Verification items for the finished model (mm, model axes). Give positions to 0.01 mm unless a question says otherwise; leave off trailing zeros. Loops run counter-clockwise (first coordinate to the right, second up) from the corner with the lowest first, then second, coordinate; pieces in that order, holes last. Notation, with made-up numbers: (48, -39.75) - (60, -39.75) arc R22 cw to (60, -30.75) - close; hole circle Ø4 at (-6.75, 1.5). An arc over 180 degrees is marked (long way). One line per question, with ' | ' between items. Start each with the question number.
1. Section check A-A, the plane z = 2.75. Enter the section's corners in (x, y).
2. Mould release check, pull along X, two halves, no side actions. Record for faces 1 (the face through (0.27, 1.22, 2.03)), 2 (the face through (4.594, -3.219, 3.512)), 3 (the face through (0, 2, 0)), 4 (the face through (-4.594, 3.219, 3.512)): +X half, -X half, draft (parallel to the pull), parting line (faces both ways), or undercut.
3. Thickness scan on line 1 along Y through (x, z) = (0, 1.45); line 2 along X through (y, z) = (0.5, 2.75); line 3 along Y through (x, z) = (-5, 1.75). Record the ranges inside material, lowest first. Write a range as from..to.
4. Section check D-D, the plane x = 3.5. Enter the section's corners in (y, z), then the cut area to 3 significant figures.
5. Section check C-C, the plane y = -1.75. Enter the section's corners in (x, z).
6. Section check B-B, the plane z = 5.75. Enter the section's corners in (x, y), then the cut area to 3 significant figures.
7. Depth check by flat-ended pin: pin 1 Ø2 at (x, y) = (0, 0) entering from -Z; pin 2 Ø1.5 at (y, z) = (2.5, 4.5) entering from +X. Enter the tip coordinate at first touch or a pass-through.
from build123d import *

# Parameters (mm, degrees)
SKETCH1_W                       = 12.7
SKETCH1_H                       = 12.7
BOSS_EXTRUDE1_DEPTH             = 6.928
TAP_DRILL_FOR_M3X0_5_TAP3_D     = 2.5
TAP_DRILL_FOR_M3X0_5_TAP3_DEPTH = 4
TAP_DRILL_FOR_M3X0_5_TAP3_TIP   = 0.751075774
CUT_EXTRUDE1_DEPTH              = 12.342053782
MIRROR2_COPY_1_DEPTH            = 12.342053782


with BuildPart() as part:
    # Sketch1 → Boss-Extrude1 (new body)
    with BuildSketch(Plane.XY):
        Rectangle(SKETCH1_W, SKETCH1_H)
    extrude(amount=BOSS_EXTRUDE1_DEPTH)

    # Tap Drill for M3x0.5 Tap3
    with Locations(Plane(origin=(0, 0, 0), x_dir=(1, 0, 0), z_dir=(0, 0, -1))):
        with Locations((0, 0)):
            Hole(TAP_DRILL_FOR_M3X0_5_TAP3_D / 2, depth=TAP_DRILL_FOR_M3X0_5_TAP3_DEPTH)
            with Locations((0, 0, -(TAP_DRILL_FOR_M3X0_5_TAP3_DEPTH + TAP_DRILL_FOR_M3X0_5_TAP3_TIP / 2))):  # 118° drill point
                Cone(0, TAP_DRILL_FOR_M3X0_5_TAP3_D / 2, TAP_DRILL_FOR_M3X0_5_TAP3_TIP, mode=Mode.SUBTRACT)

    # Sketch8 → Cut-Extrude1 (cut, symmetric)
    with BuildSketch(Plane.XY):
        Polygon((-16.943244885, 42.69979937), (2.886, 6.35), (6.35, 0), (26.179244885, -36.34979937), (98.878843624, 3.308690399), (55.756353855, 82.358289139), align=None)
    cut_extrude1 = extrude(amount=CUT_EXTRUDE1_DEPTH, both=True, mode=Mode.SUBTRACT)

    # Mirror1: Cut-Extrude1 across plane
    add(cut_extrude1.mirror(Plane.ZX), mode=Mode.SUBTRACT)

    # Mirror2: Cut-Extrude1 across plane
    add(cut_extrude1.mirror(Plane(origin=(0, 0, 0), x_dir=(0, 0, 1), z_dir=(1, 0, 0))), mode=Mode.SUBTRACT)

    # Mirror2 copy 1 sketch → Mirror2 copy 1 (cut, symmetric)
    with BuildSketch(Plane(origin=(0, 0, 0), x_dir=(-1, 0, 0), z_dir=(0, 0, 1))):
        Polygon((-16.943244885, 42.69979937), (2.886, 6.35), (6.35, 0), (26.179244885, -36.34979937), (98.878843624, 3.308690399), (55.756353855, 82.358289139), align=None)
    extrude(amount=MIRROR2_COPY_1_DEPTH, both=True, mode=Mode.SUBTRACT)


solid = part.part
Results list:
1) outline: (-6.35, 0) - (-2.89, -6.35) - (2.89, -6.35) - (6.35, 0) - (2.89, 6.35) - (-2.89, 6.35) - close; hole circle Ø2.5 at (0, 0)
2) face 1: undercut | face 2: +X half | face 3: draft | face 4: -X half
3) line 1: -6.35..-1.25, 1.25..6.35 | line 2: -6.08..-1.15, 1.15..6.08 | line 3: -2.47..2.47
4) outline: (-5.22, 0) - (5.22, 0) - (5.22, 6.93) - (-5.22, 6.93) - close | area: 72.4 mm²
5) outline: (-5.4, 0) - (5.4, 0) - (5.4, 6.93) - (-5.4, 6.93) - close
6) outline: (-6.35, 0) - (-2.89, -6.35) - (2.89, -6.35) - (6.35, 0) - (2.89, 6.35) - (-2.89, 6.35) - close | area: 117 mm²
7) pin 1: z = 4.15 | pin 2: x = 5.4
